Autodesk Inventor part; units mm, degrees
ref_plane "pin_XY" through (7.9375, 0, 0) normal (1, 0, 0) x (0, 0, -1)
ref_plane "pin_YZ" through (7.9375, 0, 0) normal (0, 0, -1) x (0, 1, 0)
ref_plane "pin_ZX" through (7.9375, 0, 0) normal (0, 1, 0) x (1, 0, 0)
sketch "Sketch_1" plane through (0, 0, 0) normal (0, 0, 1) x (1, 0, 0)
  line L0 (15.875, 0) -> (0, 0)
  line L1 (0, 0) -> (0, 1.665)
  line L2 (0, 1.665) -> (0.3048, 1.9698)
  line L3 (0.3048, 1.9698) -> (1.2192, 1.9698)
  line L4 (1.2192, 1.9698) -> (1.2192, 1.4859)
  line L5 (1.2192, 1.4859) -> (1.9812, 1.4859)
  line L6 (1.9812, 1.4859) -> (1.9812, 1.9698)
  line L7 (1.9812, 1.9698) -> (13.8938, 1.9698)
  line L8 (13.8938, 1.9698) -> (13.8938, 1.4859)
  line L9 (13.8938, 1.4859) -> (14.6558, 1.4859)
  line L10 (14.6558, 1.4859) -> (14.6558, 1.9698)
  line L11 (14.6558, 1.9698) -> (15.5702, 1.9698)
  line L12 (15.5702, 1.9698) -> (15.875, 1.665)
  line L13 (15.875, 1.665) -> (15.875, 0)
  line L14 (15.875, 0) -> (0, 0)
revolve "Revolution1" add sketch "Sketch_1" angle 360 about axis through (15.875, 0, 0) along (1, 0, 0)
ref_plane "pin_XY" through (7.9375, 0, 0) normal (1, 0, 0) x (0, 0, -1)
ref_plane "pin_YZ" through (7.9375, 0, 0) normal (0, 0, -1) x (0, 1, 0)
ref_plane "pin_ZX" through (7.9375, 0, 0) normal (0, 1, 0) x (1, 0, 0)
ref_plane "rr1_XY" through (1.6002, 0, 0) normal (1, 0, 0) x (0, 0, -1)
ref_plane "rr1_YZ" through (1.6002, 0, 0) normal (0, 0, -1) x (0, 1, 0)
ref_plane "rr1_ZX" through (1.6002, 0, 0) normal (0, 1, 0) x (1, 0, 0)
ref_plane "rr2_XY" through (14.2748, 0, 0) normal (1, 0, 0) x (0, 0, -1)
ref_plane "rr2_YZ" through (14.2748, 0, 0) normal (0, 0, -1) x (0, 1, 0)
ref_plane "rr2_ZX" through (14.2748, 0, 0) normal (0, 1, 0) x (1, 0, 0)
properties part number "D-9769-clevis_pin" material "Steel"
Input: part model. Units: mm. Frame: model coordinates. Coordinates: 2 decimals unless noted, no trailing zeros. Loops run counter-clockwise (first coordinate to the right, second up) from the corner with the lowest first, then second, coordinate; pieces in that order, holes last.
(1) Section A-A on z = 0. Return the cut outline in (x, y) (3 decimals).
(2) Section C-C on x = 8.5. Return the cut outline in (y, z), then the cut area to 3 significant figures.
(3) Pull-direction query (X, two-part tool) for faces 1 (the face through (15.119, -0.427, -1.923)), 2 (the face through (1.606, 1.417, 0.446)), 3 (the face through (14.28, 1.417, 0.446)), 4 (the face through (15.875, 0, 0)); classes: released by +X, released by -X, zero draft, split by the parting line, or undercut.
(4) First-contact query: pin 1 Ø1.5 at (x, z) = (9.5, 1) entering from -Y; pin 2 Ø2 at (x, z) = (13, -1.5) entering from +Y. Flat tips, straight axial feed; report the tip coordinate or a pass-through.
(5) Material intervals for probe 1 along X at (y, z) = (1.45, 0.7) (3 decimals); probe 2 along X at (y, z) = (-1.2, 1.3); probe 3 along Z at (x, y) = (15, 1.05), sorted ascending.
Data:
1. outline: (0, -1.665) - (0.305, -1.97) - (1.219, -1.97) - (1.219, -1.486) - (1.981, -1.486) - (1.981, -1.97) - (13.894, -1.97) - (13.894, -1.486) - (14.656, -1.486) - (14.656, -1.97) - (15.57, -1.97) - (15.875, -1.665) - (15.875, 1.665) - (15.57, 1.97) - (14.656, 1.97) - (14.656, 1.486) - (13.894, 1.486) - (13.894, 1.97) - (1.981, 1.97) - (1.981, 1.486) - (1.219, 1.486) - (1.219, 1.97) - (0.305, 1.97) - (0, 1.665) - close
2. outline: circle Ø3.94 at (0, 0)
2. area: 12.2 mm2
3. face 1: zero draft
3. face 2: undercut
3. face 3: undercut
3. face 4: released by +X
4. pin 1: stops at y = -1.95
4. pin 2: stops at y = 1.91
5. probe 1: x = 0 to 1.219, 1.981 to 13.894, 14.656 to 15.875
5. probe 2: x = 0.1 to 1.22, 1.98 to 13.89, 14.66 to 15.77
5. probe 3: z = -1.67 to 1.67
